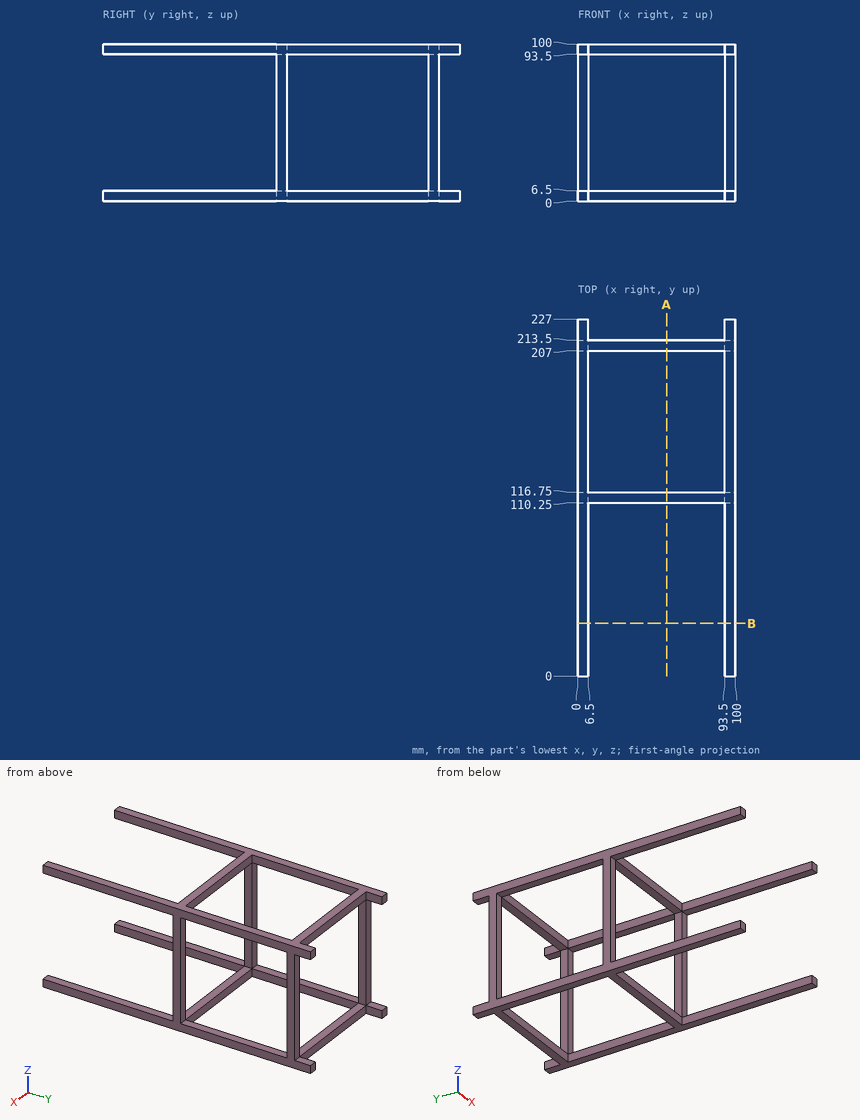
Print and shaded views of the part. All mm, measured from the part's lowest x, y and z. Coordinates: 2 decimals unless noted, no trailing zeros. Loops run counter-clockwise (first coordinate to the right, second up) from the corner with the lowest first, then second, coordinate; pieces in that order, holes last. Notation, with made-up numbers: (39, 69.25) -> (50, 69.25) arc R18 cw to (50, 84.25) -> close; hole circle Ø8 at (56, 34). An arc over 180 degrees is marked (long way). Use a Markdown table: item, result. Add a question column.
Item 1: Band-saw the part on A-A on x = 56.5. Write the cut outline in (y, z), plus the area to 3 significant figures.
Item 2: Band-saw the part on B-B on y = 33.5. Write the cut outline in (x, z), plus the area to 3 significant figures.
Item 3: Probe probe 1 along Z at (x, y) = (6, 216.5). List the from-to ranges inside material, lowest first.
Item 4: Flat gauge pins, fed straight in: P1, Ø5, axis at x = 52, z = 2, coming from the -Y side; P2, Ø2, axis at x = 2.5, z = 40, coming from the +Y side. Where does each tip first touch, or does it go through?
Geometry says:
| question | item | result |
|---|---|---|
| 1 | outline | (110.25, 0) -> (116.75, 0) -> (116.75, 6.5) -> (110.25, 6.5) -> close; (110.25, 93.5) -> (116.75, 93.5) -> (116.75, 100) -> (110.25, 100) -> close; (207, 0) -> (213.5, 0) -> (213.5, 6.5) -> (207, 6.5) -> close; (207, 93.5) -> (213.5, 93.5) -> (213.5, 100) -> (207, 100) -> close |
| 1 | area | 169 mm² |
| 2 | outline | (0, 0) -> (6.5, 0) -> (6.5, 6.5) -> (0, 6.5) -> close; (0, 93.5) -> (6.5, 93.5) -> (6.5, 100) -> (0, 100) -> close; (93.5, 0) -> (100, 0) -> (100, 6.5) -> (93.5, 6.5) -> close; (93.5, 93.5) -> (100, 93.5) -> (100, 100) -> (93.5, 100) -> close |
| 2 | area | 169 mm² |
| 3 | probe 1 | 0 to 6.5, 93.5 to 100 |
| 4 | P1 | y = 110.25 |
| 4 | P2 | y = 213.5 |
